For this review, take the finished solid that the model builds, in its own axes (mm). A direction names the side the tool comes from. Give positions to 0.01 mm unless a question says otherwise; leave off trailing zeros. Write each loop counter-clockwise with the first axis right and the second up, starting at its lowest first coordinate (ties: lowest second). Pieces come first, ordered by that corner, then holes.
1) For P1, Ø4, axis at y = -101.5, z = 14.5, coming from the +X side; P2, Ø1.5, axis at x = 33, y = 196, coming from the -Z side; P3, Ø4, axis at y = -114.5, z = 12, coming from the +X side, all flat-tipped, find the tip position at first contact; note any pin that passes through.
2) Machinability: for faces 1 (the face through (-1, -250, 14)), 2 (the face through (0, -4, 29.739)), 3 (the face through (0, -4, 28.099)), which of the approach directions +Z, -Z, +X, -X, +Y, -Y give a long, thin tool a straight path to every point of the face, cutting with its end or side? Answer none if there is none.
3) We need section B-B on x = -6.5. Give the boundary of the cut face in (y, z).
4) Wall thickness on line 1 along Z through (x, y) = (13, 81.5); line 2 along Z through (x, y) = (-4, 92.5); line 3 along X through (y, z) = (178, 17.5): over which ranges is each line inside the solid? List them lowest first.
5) We need section A-A on y = 132. Give the boundary of the cut face in (x, z).
6) We need section C-C on z = 4. Give the boundary of the cut face in (x, y), and give its area (3 significant figures).
7) We need section D-D on x = 39. Give the boundary of the cut face in (y, z).
8) Draft analysis for pull direction X (two halves, no side actions). For faces 4 (the face through (0, -4, 15.099)), 5 (the face through (-34, -4, 31.039)), 6 (the face through (-19, -4, 22)), 7 (the face through (-40.869, -3.5, 7.437)), state which applies: pulls with the +X half, pulls with the -X half, needs draft (parallel to the pull), parting line crosses it, or undercut.
from build123d import *

# Parameters (mm, degrees)
F1_DEPTH    = 250
F2_R        = 5
F3_R        = 1
F4_W        = 38
F4_H        = 13
F5_DEPTH    = 500.001
F6_T1_DEPTH = 509.3674969976


# Not quite as in the source:
# - a fillet or chamfer that OpenCascade refuses, or shapes differently, is made with other operations: its cross-section is extruded or revolved along the edge and cut away or added


with BuildPart() as f1:
    # F0 (on Front) → F1 (new body, symmetric)
    with BuildSketch(Plane.XZ):
        with BuildLine():
            Line((22.5, 29.7386717319), (0, 29.7386717319))
            Line((0, 29.7386717319), (-22.5, 29.7386717319))
            Line((-22.5, 29.7386717319), (-22.5, 31.0386717319))
            Line((-22.5, 31.0386717319), (-45.5824640741, 31.0386717319))
            Line((-45.5824640741, 31.0386717319), (-57.5, 21.0386717319))
            Line((-57.5, 21.0386717319), (-57.5, 17.0386717319))
            Line((-57.5, 17.0386717319), (-22.8589838486, -2.9613282681))
            ThreePointArc((-22.8589838486, -2.9613282681), (0, -1.6507010523), (22.8589838486, -2.9613282681))
            Line((22.8589838486, -2.9613282681), (57.5, 17.0386717319))
            Line((57.5, 17.0386717319), (57.5, 21.0386717319))
            Line((57.5, 21.0386717319), (45.5824640741, 31.0386717319))
            Line((45.5824640741, 31.0386717319), (22.5, 31.0386717319))
            Line((22.5, 31.0386717319), (22.5, 29.7386717319))
        make_face()
    extrude(amount=F1_DEPTH, both=True)

    # F2
    f2_edges = [f1.edges().sort_by_distance(p)[0] for p in [
        (45.582464, 0, 31.038672),
        (22.858984, 0, -2.961328),
        (-45.582464, 0, 31.038672),
        (-22.858984, 0, -2.961328),
    ]]
    fillet(f2_edges, radius=F2_R)

    # F3
    f3_edges = [f1.edges().sort_by_distance(p)[0] for p in [
        (57.5, 0, 21.038672),
        (57.5, 0, 17.038672),
        (-57.5, 0, 21.038672),
        (-57.5, 0, 17.038672),
    ]]
    fillet(f3_edges, radius=F3_R)

    # F4 (on face) → F5 (cut, through all)
    with BuildSketch(Plane.XZ.offset(250)):
        with Locations((0, 21.5986846235)):
            Rectangle(F4_W, F4_H)
    extrude(amount=-F5_DEPTH, mode=Mode.SUBTRACT)

    # F6: fillet of radius 2 on 2 edges, made by hand

    # F6_s2 → F6_t1 (cut)
    with BuildSketch(Plane.XZ.offset(-254.6837484988)):
        with BuildLine():
            ThreePointArc((-22.5, 29.7386717319), (-23.2333239744, 30.6818394045), (-24.3734993995, 31.0386717319))
            Line((-24.3734993995, 31.0386717319), (-22.5, 31.0386717319))
            Line((-22.5, 31.0386717319), (-22.5, 29.7386717319))
        make_face()
        with BuildLine():
            ThreePointArc((24.3734993995, 31.0386717319), (23.2333239744, 30.6818394045), (22.5, 29.7386717319))
            Line((22.5, 29.7386717319), (22.5, 31.0386717319))
            Line((22.5, 31.0386717319), (24.3734993995, 31.0386717319))
        make_face()
    extrude(amount=F6_T1_DEPTH, mode=Mode.SUBTRACT)


solid = f1.part
Results list:
1. P1: stops at x = 56.57
1. P2: stops at z = 2.46
1. P3: stops at x = 52.24
2. face 1: +Z, -Z, +X, -X, -Y
2. face 2: +Z, +Y, -Y
2. face 3: +Y, -Y
3. outline: (-250, -1.76) - (250, -1.76) - (250, 15.1) - (-250, 15.1) - close; (-250, 28.1) - (250, 28.1) - (250, 29.74) - (-250, 29.74) - close
4. line 1: z = -2.07 to 15.1, 28.1 to 29.74
4. line 2: z = -1.69 to 15.1, 28.1 to 29.74
4. line 3: x = -57.49 to -19, 19 to 57.49
5. outline: (-57.5, 17.62) arc R1 ccw to (-57, 16.75) - (-24.28, -2.14) arc R5 ccw to (-21.25, -2.78) arc R200 cw to (21.25, -2.78) arc R5 ccw to (24.28, -2.14) - (57, 16.75) arc R1 ccw to (57.5, 17.62) - (57.5, 20.57) arc R1 ccw to (57.14, 21.34) - (46.98, 29.87) arc R5 ccw to (43.76, 31.04) - (24.37, 31.04) arc R2 ccw to (22.5, 29.74) - (-22.5, 29.74) arc R2 ccw to (-24.37, 31.04) - (-43.76, 31.04) arc R5 ccw to (-46.98, 29.87) - (-57.14, 21.34) arc R1 ccw to (-57.5, 20.57) - close; hole (-19, 15.1) - (19, 15.1) - (19, 28.1) - (-19, 28.1) - close
6. outline: (-34.92, -250) - (34.92, -250) - (34.92, 250) - (-34.92, 250) - close
6. area: 34,900 mm2
7. outline: (-250, 6.36) - (250, 6.36) - (250, 31.04) - (-250, 31.04) - close
8. face 4: undercut
8. face 5: needs draft
8. face 6: undercut
8. face 7: pulls with the -X half
